```python
from build123d import *

# Parameters (mm, degrees)
F0_R     = 1.5
F1_DEPTH = 1.5


with BuildPart() as f1:
    # F0 (on Top) → F1 (new body, symmetric)
    with BuildSketch(Plane.XY):
        Polygon((9.39682, 26.276459), (9.396826, 3.276474), (19.396826, 3.276474), (19.396826, 6.276474), (22.396826, 6.276474), (22.396826, 25.276474), (36.396826, 25.276474), (36.396826, 67.276474), (22.396826, 67.276474), (22.396826, 86.276474), (19.396826, 86.276474), (19.396826, 89.276474), (9.396826, 89.276474), (9.396826, 66.276474), (-1.603174, 66.276474), (-1.603197, 26.276459), align=None)
        with BuildLine():
            ThreePointArc((12.646826, 10.276474), (11.939719, 10.569367), (11.646826, 11.276474))
            ThreePointArc((11.646826, 11.276474), (11.939719, 11.983581), (12.646826, 12.276474))
            Line((12.646826, 12.276474), (14.146826, 12.276474))
            ThreePointArc((14.146826, 12.276474), (14.853933, 11.983581), (15.146826, 11.276474))
            ThreePointArc((15.146826, 11.276474), (14.853933, 10.569367), (14.146826, 10.276474))
            Line((14.146826, 10.276474), (12.646826, 10.276474))
        make_face(mode=Mode.SUBTRACT)
        with BuildLine():
            ThreePointArc((12.646826, 20.276474), (11.939719, 20.569367), (11.646826, 21.276474))
            ThreePointArc((11.646826, 21.276474), (11.939719, 21.983581), (12.646826, 22.276474))
            Line((12.646826, 22.276474), (14.146826, 22.276474))
            ThreePointArc((14.146826, 22.276474), (14.853933, 21.983581), (15.146826, 21.276474))
            ThreePointArc((15.146826, 21.276474), (14.853933, 20.569367), (14.146826, 20.276474))
            Line((14.146826, 20.276474), (12.646826, 20.276474))
        make_face(mode=Mode.SUBTRACT)
        with BuildLine():
            ThreePointArc((1.646826, 30.276474), (0.939719, 30.569367), (0.646826, 31.276474))
            ThreePointArc((0.646826, 31.276474), (0.939719, 31.983581), (1.646826, 32.276474))
            Line((1.646826, 32.276474), (3.146826, 32.276474))
            ThreePointArc((3.146826, 32.276474), (3.853933, 31.983581), (4.146826, 31.276474))
            ThreePointArc((4.146826, 31.276474), (3.853933, 30.569367), (3.146826, 30.276474))
            Line((3.146826, 30.276474), (1.646826, 30.276474))
        make_face(mode=Mode.SUBTRACT)
        with BuildLine():
            ThreePointArc((1.646826, 40.276474), (0.939719, 40.569367), (0.646826, 41.276474))
            ThreePointArc((0.646826, 41.276474), (0.939719, 41.983581), (1.646826, 42.276474))
            Line((1.646826, 42.276474), (3.146826, 42.276474))
            ThreePointArc((3.146826, 42.276474), (3.853933, 41.983581), (4.146826, 41.276474))
            ThreePointArc((4.146826, 41.276474), (3.853933, 40.569367), (3.146826, 40.276474))
            Line((3.146826, 40.276474), (1.646826, 40.276474))
        make_face(mode=Mode.SUBTRACT)
        with Locations((29.896826, 34.276474)):
            Circle(F0_R, mode=Mode.SUBTRACT)
        with BuildLine():
            ThreePointArc((1.646826, 50.276474), (0.939719, 50.569367), (0.646826, 51.276474))
            ThreePointArc((0.646826, 51.276474), (0.939719, 51.983581), (1.646826, 52.276474))
            Line((1.646826, 52.276474), (3.146826, 52.276474))
            ThreePointArc((3.146826, 52.276474), (3.853933, 51.983581), (4.146826, 51.276474))
            ThreePointArc((4.146826, 51.276474), (3.853933, 50.569367), (3.146826, 50.276474))
            Line((3.146826, 50.276474), (1.646826, 50.276474))
        make_face(mode=Mode.SUBTRACT)
        with BuildLine():
            ThreePointArc((1.646826, 60.276474), (0.939719, 60.569367), (0.646826, 61.276474))
            ThreePointArc((0.646826, 61.276474), (0.939719, 61.983581), (1.646826, 62.276474))
            Line((1.646826, 62.276474), (3.146826, 62.276474))
            ThreePointArc((3.146826, 62.276474), (3.853933, 61.983581), (4.146826, 61.276474))
            ThreePointArc((4.146826, 61.276474), (3.853933, 60.569367), (3.146826, 60.276474))
            Line((3.146826, 60.276474), (1.646826, 60.276474))
        make_face(mode=Mode.SUBTRACT)
        with BuildLine():
            ThreePointArc((12.646826, 70.276474), (11.939719, 70.569367), (11.646826, 71.276474))
            ThreePointArc((11.646826, 71.276474), (11.939719, 71.983581), (12.646826, 72.276474))
            Line((12.646826, 72.276474), (14.146826, 72.276474))
            ThreePointArc((14.146826, 72.276474), (14.853933, 71.983581), (15.146826, 71.276474))
            ThreePointArc((15.146826, 71.276474), (14.853933, 70.569367), (14.146826, 70.276474))
            Line((14.146826, 70.276474), (12.646826, 70.276474))
        make_face(mode=Mode.SUBTRACT)
        with BuildLine():
            ThreePointArc((12.646826, 80.276474), (11.939719, 80.569367), (11.646826, 81.276474))
            ThreePointArc((11.646826, 81.276474), (11.939719, 81.983581), (12.646826, 82.276474))
            Line((12.646826, 82.276474), (14.146826, 82.276474))
            ThreePointArc((14.146826, 82.276474), (14.853933, 81.983581), (15.146826, 81.276474))
            ThreePointArc((15.146826, 81.276474), (14.853933, 80.569367), (14.146826, 80.276474))
            Line((14.146826, 80.276474), (12.646826, 80.276474))
        make_face(mode=Mode.SUBTRACT)
        with Locations((29.896826, 58.276474)):
            Circle(F0_R, mode=Mode.SUBTRACT)
    extrude(amount=F1_DEPTH, both=True)


solid = f1.part
```
Build history of the part. All positions in model axes, mm. A direction names the side the tool comes from. Round coordinates to 2 decimals unless told otherwise and drop trailing zeros. Order: outer loops, then holes, each group sorted by start corner. A loop starts at its lowest first (then second) coordinate and runs counter-clockwise, first axis right, second up. Notation, with made-up numbers: (0.25, 40) -> (26.25, 40) arc R35 ccw to (26.25, 78) -> close; hole circle Ø5 at (8.25, -12). An arc over 180 degrees is marked (long way). Answer in a Markdown table with one row per item.
1) Pin check, flat tips, straight feed: P1, Ø3.5, axis at x = 29.9, y = 58.28, coming from the -Z side; P2, Ø1.6, axis at x = 2.5, z = 0, coming from the -Y side; P3, Ø1.5, axis at y = 74.5, z = -0.5, coming from the +X side; P4, Ø0.9, axis at y = 14, z = 0.5, coming from the -X side. Stop position of each tip, or through.
Values:
| item | result |
|---|---|
| P1 | z = -1.5 |
| P2 | y = 26.28 |
| P3 | x = 22.4 |
| P4 | x = 9.4 |
2) Which spindle directions (+Z, -Z, +X, -X, +Y, -Y) get a long thin tool onto all of the face, cutting with end or side? Do faces 1 (the flat face through (17, 47, -1.5)), 2 (the flat face through (2, 42.276, 0)), 3 (the flat face through (9.397, 15, 0)), 4 (the flat face through (29, 25.276, 0)). Say none if no direction does.
Values:
| item | result |
|---|---|
| face 1 | -Z, +X, -X, +Y, -Y |
| face 2 | +Z, -Z |
| face 3 | +Z, -Z, -X, -Y |
| face 4 | +Z, -Z, +X, -Y |
3) Band-saw the part on C-C on z = -0.8. Give the number of separate pieces and of enclosed holes in the cut face, and give its area (3 significant figures).
Values:
| item | result |
|---|---|
| separate pieces | 1 |
| enclosed holes | 10 |
| area | 2,060 mm2 |
4) Band-saw the part on A-A on x = 21. Give the cut face in (y, z).
Values:
| item | result |
|---|---|
| outline | (6.28, -1.5) -> (86.28, -1.5) -> (86.28, 1.5) -> (6.28, 1.5) -> close |
5) Band-saw the part on B-B on y = 17.5. Give the cut face in (x, z).
Values:
| item | result |
|---|---|
| outline | (9.4, -1.5) -> (22.4, -1.5) -> (22.4, 1.5) -> (9.4, 1.5) -> close |
6) Mould opens along Y. For faces 5 (the flat face through (14, 3.276, 0)), 6 (the flat face through (22.397, 16, 0)), 7 (the flat face through (13, 12.276, 0)) say: released by +Y, released by -Y, zero draft, split by the parting line, or undercut.
Values:
| item | result |
|---|---|
| face 5 | released by -Y |
| face 6 | zero draft |
| face 7 | undercut |
7) Wall check: L1, parallel to Y at x = 2.5, z = -0.7; L2, parallel to Y at x = 13, z = -1.05; L3, parallel to Y at x = 31, z = -1.1. Give the ranges that are in metal, low to high.
Values:
| item | result |
|---|---|
| L1 | 26.28 to 30.28, 32.28 to 40.28, 42.28 to 50.28, 52.28 to 60.28, 62.28 to 66.28 |
| L2 | 3.28 to 10.28, 12.28 to 20.28, 22.28 to 70.28, 72.28 to 80.28, 82.28 to 89.28 |
| L3 | 25.28 to 33.26, 35.29 to 57.26, 59.29 to 67.28 |
